from build123d import *

# Parameters (mm, degrees)
AUFSATZ_LINEAR_AUSTRAGEN1_DEPTH      = 3
AUFSATZ_LINEAR_AUSTRAGEN1_DEPTH_BACK = 1
AUFSATZ_LINEAR_AUSTRAGEN3_DEPTH      = 31.65
SKIZZE7_R                            = 2.5
SCHNITT_LINEAR_AUSTRAGEN2_DEPTH      = 110.867294952
SCHNITT_LINEAR_AUSTRAGEN6_DEPTH      = 2
SKIZZE10_R                           = 1.25
SCHNITT_LINEAR_AUSTRAGEN7_DEPTH      = 111.405717696
SKIZZE11_R                           = 2.75
SCHNITT_LINEAR_AUSTRAGEN8_DEPTH      = 1.4
SKIZZE14_R                           = 1.05
SCHNITT_LINEAR_AUSTRAGEN9_DEPTH      = 10
SKIZZE15_R                           = 1.75
AUFSATZ_LINEAR_AUSTRAGEN4_DEPTH      = 16
SKIZZE16_R                           = 0.65
AUFSATZ_LINEAR_AUSTRAGEN5_DEPTH      = 2
SKIZZE18_R                           = 1.1
SCHNITT_LINEAR_AUSTRAGEN10_DEPTH     = 13


with BuildPart() as part:
    # Skizze2 → Aufsatz-Linear austragen1 (new, two sides: drawn at the far end of the back side and taken through both)
    with BuildSketch(Plane(origin=(0, 0, 0), x_dir=(1, 0, 0), z_dir=(0, 1, 0)).offset(-AUFSATZ_LINEAR_AUSTRAGEN1_DEPTH_BACK)):
        Polygon((-53.033008589, 53.033008589), (0, 0), (53.033008589, 53.033008589), (0, 75), align=None)
        Polygon((53.033008589, 53.033008589), (0, 0), (75, 0), align=None)
        Polygon((75, 0), (0, 0), (53.033008589, -53.033008589), align=None)
        Polygon((53.033008589, -53.033008589), (0, 0), (-53.033008589, -53.033008589), (0, -75), align=None)
        Polygon((-53.033008589, 53.033008589), (-75, 0), (0, 0), align=None)
        Polygon((0, 0), (-75, 0), (-53.033008589, -53.033008589), align=None)
    extrude(amount=AUFSATZ_LINEAR_AUSTRAGEN1_DEPTH + AUFSATZ_LINEAR_AUSTRAGEN1_DEPTH_BACK)

    # Skizze5 → Aufsatz-Linear austragen3 (add)
    with BuildSketch(Plane(origin=(0, 0, 0), x_dir=(1, 0, 0), z_dir=(0, 1, 0))):
        Polygon((-4, 18.306991411), (-4, 10.306991411), (-10.335850601, 10.306991411), (-10.335850601, -30.593008589), (9.764149399, -30.593008589), (9.764149399, 10.306991411), (4, 10.306991411), (4, 18.306991411), (11.764149399, 18.306991411), (11.764149399, -38.593008589), (-12.185850601, -38.593008589), (-12.185850601, 18.306991411), align=None)
    extrude(amount=AUFSATZ_LINEAR_AUSTRAGEN3_DEPTH)

    # Skizze7 → Schnitt-Linear austragen2 (cut, through all)
    with BuildSketch(Plane(origin=(0, 3, 0), x_dir=(1, 0, 0), z_dir=(0, 1, 0))):
        with Locations(Location((35, 40, 0), (0, 0, 270))):
            Circle(SKIZZE7_R)
        with Locations(Location((-35, 40, 0), (0, 0, 270))):
            Circle(SKIZZE7_R)
        with Locations(Location((0, -50, 0), (0, 0, 270))):
            Circle(SKIZZE7_R)
    extrude(amount=-SCHNITT_LINEAR_AUSTRAGEN2_DEPTH, mode=Mode.SUBTRACT)

    # Skizze8 → Schnitt-Linear austragen6 (cut)
    with BuildSketch(Plane(origin=(0, 3, 0), x_dir=(1, 0, 0), z_dir=(0, 1, 0))):
        Polygon((-22, 8.05), (-22, -8.05), (-39.6, 0), align=None)
        Polygon((22, -8.05), (39.6, 0), (22, 8.05), align=None)
    extrude(amount=-SCHNITT_LINEAR_AUSTRAGEN6_DEPTH, mode=Mode.SUBTRACT)

    # Skizze10 → Schnitt-Linear austragen7 (cut, through all)
    with BuildSketch(Plane(origin=(0, 1, 0), x_dir=(1, 0, 0), z_dir=(0, 1, 0))):
        with Locations(Location((-27.087800905, -51.780869351, 0), (0, 0, 270))):
            Circle(SKIZZE10_R)
        with Locations(Location((27.09, 0.05, 0), (0, 0, 90))):
            Circle(SKIZZE10_R)
    extrude(amount=-SCHNITT_LINEAR_AUSTRAGEN7_DEPTH, mode=Mode.SUBTRACT)

    # Skizze11 → Schnitt-Linear austragen8 (cut)
    with BuildSketch(Plane.XZ.offset(1)):
        with Locations(Location((-27.087800905, 51.780869351, 0), (0, 0, 270))):
            Circle(SKIZZE11_R)
        with Locations(Location((27.09, -0.05, 0), (0, 0, 270))):
            Circle(SKIZZE11_R)
    extrude(amount=-SCHNITT_LINEAR_AUSTRAGEN8_DEPTH, mode=Mode.SUBTRACT)

    # Skizze14 → Schnitt-Linear austragen9 (cut)
    with BuildSketch(Plane(origin=(0, 3, 0), x_dir=(1, 0, 0), z_dir=(0, 1, 0))):
        with Locations(Location((-58.5, 0, 0), (0, 0, 270))):
            Circle(SKIZZE14_R)
        with Locations(Location((-41.365746699, 41.365746699, 0), (0, 0, 270))):
            Circle(SKIZZE14_R)
        with Locations(Location((41.365746699, 41.365746699, 0), (0, 0, 270))):
            Circle(SKIZZE14_R)
        with Locations(Location((58.5, 0, 0), (0, 0, 270))):
            Circle(SKIZZE14_R)
        with Locations(Location((41.365746699, -41.365746699, 0), (0, 0, 270))):
            Circle(SKIZZE14_R)
        with Locations(Location((-41.365746699, -41.365746699, 0), (0, 0, 270))):
            Circle(SKIZZE14_R)
        with Locations(Location((0, -58.5, 0), (0, 0, 270))):
            Circle(SKIZZE14_R)
    extrude(amount=-SCHNITT_LINEAR_AUSTRAGEN9_DEPTH, mode=Mode.SUBTRACT)

    # Skizze15 → Aufsatz-Linear austragen4 (add)
    with BuildSketch(Plane(origin=(0, 3, 0), x_dir=(1, 0, 0), z_dir=(0, 1, 0))):
        with BuildLine():
            ThreePointArc((18.61, 37.536991411), (19.122563133, 36.299554544), (20.36, 35.786991411))
            Line((20.36, 35.786991411), (20.36, 37.536991411))
            Line((20.36, 37.536991411), (18.61, 37.536991411))
        make_face()
        with BuildLine():
            Line((20.36, 37.536991411), (20.36, 35.786991411))
            ThreePointArc((20.36, 35.786991411), (21.597436867, 36.299554544), (22.11, 37.536991411))
            ThreePointArc((22.11, 37.536991411), (20.36, 39.286991411), (18.61, 37.536991411))
            Line((18.61, 37.536991411), (20.36, 37.536991411))
        make_face()
        with BuildLine():
            Line((-20.36, 24.056991411), (-20.36, 22.306991411))
            Line((-20.36, 22.306991411), (-18.61, 22.306991411))
            ThreePointArc((-18.61, 22.306991411), (-19.122563133, 23.544428278), (-20.36, 24.056991411))
        make_face()
        with BuildLine():
            Line((-18.61, 22.306991411), (-20.36, 22.306991411))
            Line((-20.36, 22.306991411), (-20.36, 24.056991411))
            ThreePointArc((-20.36, 24.056991411), (-21.597436867, 21.069554544), (-18.61, 22.306991411))
        make_face()
        with BuildLine():
            ThreePointArc((-18.61, 37.536991411), (-21.597436867, 38.774428278), (-20.36, 35.786991411))
            Line((-20.36, 35.786991411), (-20.36, 37.536991411))
            Line((-20.36, 37.536991411), (-18.61, 37.536991411))
        make_face()
        with BuildLine():
            Line((-20.36, 37.536991411), (-20.36, 35.786991411))
            ThreePointArc((-20.36, 35.786991411), (-19.122563133, 36.299554544), (-18.61, 37.536991411))
            Line((-18.61, 37.536991411), (-20.36, 37.536991411))
        make_face()
        with Locations(Location((20.36, 22.306991411, 0), (0, 0, 270))):
            Circle(SKIZZE15_R)
    extrude(amount=AUFSATZ_LINEAR_AUSTRAGEN4_DEPTH)

    # Skizze16 → Aufsatz-Linear austragen5 (add)
    with BuildSketch(Plane(origin=(0, 19, 0), x_dir=(1, 0, 0), z_dir=(0, 1, 0))):
        with Locations(Location((20.36, 22.306991411, 0), (0, 0, 270))):
            Circle(SKIZZE16_R)
        with Locations(Location((20.36, 37.536991411, 0), (0, 0, 270))):
            Circle(SKIZZE16_R)
        with Locations(Location((-20.36, 37.536991411, 0), (0, 0, 270))):
            Circle(SKIZZE16_R)
        with Locations(Location((-20.36, 22.306991411, 0), (0, 0, 270))):
            Circle(SKIZZE16_R)
    extrude(amount=AUFSATZ_LINEAR_AUSTRAGEN5_DEPTH)

    # Skizze18 → Schnitt-Linear austragen10 (cut)
    with BuildSketch(Plane(origin=(0, 31.65, 0), x_dir=(1, 0, 0), z_dir=(0, 1, 0))):
        with Locations(Location((-5.785850601, 14.856991411, 0), (0, 0, 270))):
            Circle(SKIZZE18_R)
        with Locations(Location((5.5, 14.856991411, 0), (0, 0, 270))):
            Circle(SKIZZE18_R)
        with Locations(Location((5.114149399, -34.443008589, 0), (0, 0, 270))):
            Circle(SKIZZE18_R)
        with Locations(Location((-5.785850601, -34.443008589, 0), (0, 0, 270))):
            Circle(SKIZZE18_R)
    extrude(amount=-SCHNITT_LINEAR_AUSTRAGEN10_DEPTH, mode=Mode.SUBTRACT)


solid = part.part
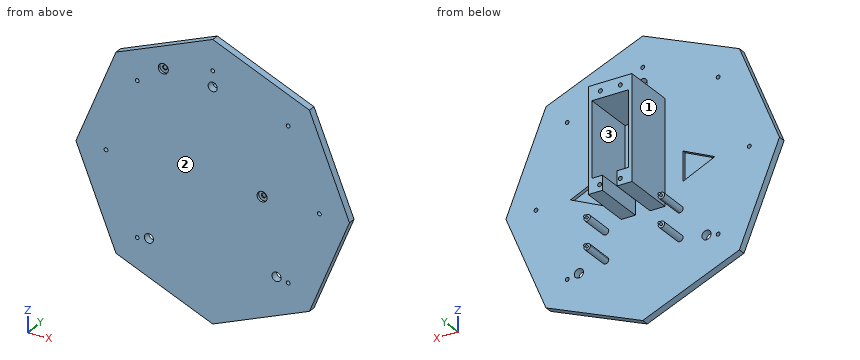
Could you check a few things on this model? Use its own coordinates, in mm. Face numbers are marked on the shaded views. A direction names the side the tool comes from. Round coordinates to 2 decimals unless told otherwise and drop trailing zeros. Write each loop counter-clockwise with the first axis right and the second up, starting at its lowest first coordinate (ties: lowest second). Pieces come first, ordered by that corner, then holes. Notation, with made-up numbers: (18.5, -9) -> (68.5, -9) arc R14 ccw to (68.5, 7) -> close; hole circle Ø7 at (14, 50.25). An arc over 180 degrees is marked (long way). Use a Markdown table: item, result.
1. If we section it at C-C (z = -6): List the corners of the cut face in (x, y) for me.
Answer key:
| item | result |
|---|---|
| outline | (-72.51, -1) -> (72.51, -1) -> (72.51, 3) -> (26.48, 3) -> (26.48, 1) -> (22, 1) -> (22, 3) -> (11.76, 3) -> (11.76, 31.65) -> (9.76, 31.65) -> (9.76, 3) -> (-10.34, 3) -> (-10.34, 31.65) -> (-12.19, 31.65) -> (-12.19, 3) -> (-22, 3) -> (-22, 1) -> (-26.48, 1) -> (-26.48, 3) -> (-72.51, 3) -> close |
2. If we section it at B-B (y = 23): List the corners of the cut face in (x, z) for me.
Answer key:
| item | result |
|---|---|
| outline | (-12.19, -18.31) -> (-4, -18.31) -> (-4, -10.31) -> (-10.34, -10.31) -> (-10.34, 30.59) -> (9.76, 30.59) -> (9.76, -10.31) -> (4, -10.31) -> (4, -18.31) -> (11.76, -18.31) -> (11.76, 38.59) -> (-12.19, 38.59) -> close; hole circle Ø2.2 at (-5.79, -14.86); hole circle Ø2.2 at (-5.79, 34.44); hole circle Ø2.2 at (5.11, 34.44); hole circle Ø2.2 at (5.5, -14.86) |
3. Please list where these lines run through material, in increasing order: probe 1 along X at (y, z) = (8, -13); probe 2 along X at (y, z) = (0, 0); probe 3 along Z at (x, y) = (8.5, 25.5).
Answer key:
| item | result |
|---|---|
| probe 1 | x = -12.19 to -4, 4 to 11.76 |
| probe 2 | x = -75 to -59.55, -57.45 to 24.34, 29.84 to 57.45, 59.55 to 75 |
| probe 3 | z = -18.31 to -10.31, 30.59 to 38.59 |
4. For pin 1 Ø6.5 at (y, z) = (21, -15) entering from +X; pin 2 Ø6 at (x, y) = (-2.5, 14) entering from -Z; pin 3 Ø5 at (x, z) = (-27.09, 51.78) entering from +Y; pin 4 Ø1.7 at (x, z) = (0, 58.5) entering from -Y, each with a flat end and sliding along its axis, tell me the tip position at first contact or that it passes through.
Answer key:
| item | result |
|---|---|
| pin 1 | stops at x = 11.76 |
| pin 2 | stops at z = -18.31 |
| pin 3 | stops at y = 3 |
| pin 4 | passes through |
5. Which directions (+Z, -Z, +X, -X, +Y, -Y) give clear straight access to the entire face, cutting with the end or side of a thin tool? Please do the marked faces 1, 2 and 3.
Answer key:
| item | result |
|---|---|
| face 1 | +Z, -Z, -X, +Y |
| face 2 | +Z, -Z, +X, -X, -Y |
| face 3 | +Y |
6. If we section it at A-A (y = 13): List the corners of the cut face in (x, z) for me.
Answer key:
| item | result |
|---|---|
| outline | circle Ø3.5 at (-20.36, -37.54); circle Ø3.5 at (-20.36, -22.31); (-12.19, -18.31) -> (-4, -18.31) -> (-4, -10.31) -> (-10.34, -10.31) -> (-10.34, 30.59) -> (9.76, 30.59) -> (9.76, -10.31) -> (4, -10.31) -> (4, -18.31) -> (11.76, -18.31) -> (11.76, 38.59) -> (-12.19, 38.59) -> close; circle Ø3.5 at (20.36, -37.54); circle Ø3.5 at (20.36, -22.31) |
7. If we section it at D-D (x = -51): List the corners of the cut face in (y, z) for me, then the cut area to 3 significant figures.
Answer key:
| item | result |
|---|---|
| outline | (-1, -53.88) -> (3, -53.88) -> (3, 53.88) -> (-1, 53.88) -> close |
| area | 431 mm^2 |
